Read the model definition and answer for the solid it produces. Units are mm, in the model's axes. Give positions to 0.01 mm unless a question says otherwise; leave off trailing zeros. Order: outer loops, then holes, each group sorted by start corner. A loop starts at its lowest first (then second) coordinate and runs counter-clockwise, first axis right, second up. Notation, with made-up numbers: (21.5, 76) -> (38.5, 76) arc R20 cw to (38.5, 94) -> close; hole circle Ø5 at (-17.5, -37). An arc over 180 degrees is marked (long way). One line per question, with ' | ' between items. Start each with the question number.
Autodesk Inventor part; units mm, degrees
ref_plane "Work Plane1" through (0, 0, 4) normal (0, 0, 1) x (1, 0, 0)
ref_plane "Work Plane3" through (0, 0, -1) normal (0, 0, 1) x (1, 0, 0)
ref_plane "Work Plane4" through (0, 0, 0) normal (0, 0, -1) x (-1, 0, 0)
sketch "Sketch1" plane through (0, 0, 0) normal (0, 0, 1) x (1, 0, 0)
  circle A0 centre (0, 0) radius 55
  dimension "d0" = 110
extrude "Extrusion1" add sketch "Sketch1" along normal blind 3
ref_plane "Work Plane1" through (0, 0, 4) normal (0, 0, 1) x (1, 0, 0)
sketch "Sketch2" plane through (0, 0, 4) normal (0, 0, 1) x (1, 0, 0)
  line L0 (-6.5, 6) -> (6.5, 6)
  line L1 (6.5, 6) -> (6.5, -18)
  line L2 (-6.5, -18) -> (-6.5, 6)
  circle A0 centre (-35.532, 35.532) radius 1.5
  circle A1 centre (-35.532, -35.532) radius 1.5
  circle A2 centre (35.532, -35.532) radius 1.5
  circle A3 centre (35.532, 35.532) radius 1.5
  line L3 (-6.5, -18) -> (6.5, -18)
  circle A4 centre (0, 8.5) radius 1
  circle A5 centre (0, -19.528) radius 1.9565
  point P0 (0, 0)
  point P1 (0, 6)
  point P2 (0, -13.848)
  dimension "d4" = 13
  dimension "d7" = 3
  dimension "d8" = 3
  dimension "d9" = 3
  dimension "d10" = 3
  dimension "d15" = 35.532
  dimension "d16" = 35.532
  dimension "d17" = 35.532
  dimension "d18" = 35.532
  dimension "d19" = 35.532
  dimension "d20" = 35.532
  dimension "d21" = 35.532
  dimension "d22" = 35.532
  dimension "d138" = 6
  dimension "d139" = 24
  dimension "d140" = 2
  dimension "d141" = 2.5
  dimension "d142" = 1.528
extrude "Extrusion2" cut sketch "Sketch2" against normal blind 4 contours L0 L1 L3 A5 L2 | A5 L3 picked at (0, -17.8572)
ref_plane "Work Plane2" through (0, 0, 3) normal (0, 0, 1) x (1, 0, 0)
sketch "Sketch3" plane through (0, 0, 3) normal (0, 0, 1) x (1, 0, 0)
  circle A0 centre (-35.577, 35.5342) radius 2.5
  circle A1 centre (-35.5225, -35.5931) radius 2.5
  circle A2 centre (35.5095, -35.5931) radius 2.5
  circle A3 centre (35.5095, 35.4262) radius 2.5
  point P0 (0, 0)
ref_plane "Work Plane3" through (0, 0, -1) normal (0, 0, 1) x (1, 0, 0)
ref_plane "Work Plane4" through (0, 0, 0) normal (0, 0, -1) x (-1, 0, 0)
sketch "Sketch5" plane through (0, 0, 0) normal (0, 0, -1) x (-1, 0, 0)
  line L0 (-9.906, 9.652) -> (9.906, 9.652)
  line L1 (9.906, 9.652) -> (9.906, -30.226)
  line L2 (9.906, -30.226) -> (-9.906, -30.226)
  line L3 (-9.906, -30.226) -> (-9.906, 9.652)
  circle A0 centre (-35.532, 35.532) radius 1.5
  circle A1 centre (-35.532, -35.532) radius 1.5
  circle A2 centre (35.532, -35.532) radius 1.5
  circle A3 centre (35.532, 35.532) radius 1.5
  circle A4 centre (-5.08, 13.462) radius 1
  circle A5 centre (5.08, 13.462) radius 1
  circle A6 centre (-5.08, -34.036) radius 1
  circle A7 centre (5.08, -34.036) radius 1
  point P0 (0, 0)
  point P1 (0, 0)
  point P2 (0, 9.652)
  point P3 (0, -30.226)
  dimension "d53" = 19.812
  dimension "d54" = 39.878
  dimension "d55" = 9.652
  dimension "d56" = 3
  dimension "d57" = 3
  dimension "d58" = 3
  dimension "d59" = 3
  dimension "d60" = 2
  dimension "d61" = 2
  dimension "d62" = 2
  dimension "d63" = 2
  dimension "d64" = 35.532
  dimension "d65" = 35.532
  dimension "d66" = 35.532
  dimension "d67" = 35.532
  dimension "d68" = 35.532
  dimension "d69" = 35.532
  dimension "d70" = 35.532
  dimension "d71" = 35.532
  dimension "d72" = 10.16
  dimension "d73" = 10.16
  dimension "d74" = 3.81
  dimension "d75" = 3.81
  dimension "d76" = 3.81
  dimension "d77" = 3.81
  dimension "d78" = 30.226
  dimension "d79" = 5.08
  dimension "d80" = 5.08
  dimension "d81" = 5.08
  dimension "d82" = 5.08
hole "Hole1" at (35.532, 35.532, 0) at (-35.532, 35.532, 0) at (35.532, -35.532, 0) at (-35.532, -35.532, 0) direction (0, 0, 1) diameter 2.459 depth 4 tip angle 118
ref_plane "Work Plane5" through (0, 0, 0) normal (0, 0, -1) x (-1, 0, 0)
fillet "Fillet1" radius 0.4125 4 edges at (6.5, -18, 1.5) (-6.5, -18, 1.5) (6.5, 6, 1.5) (-6.5, 6, 1.5)
ref_plane "Work Plane6" through (0, 0, 0) normal (0, 0, -1) x (-1, 0, 0)
ref_plane "Work Plane7" through (0, 0, 3) normal (0, 0, 1) x (1, 0, 0)
sketch "Sketch8" plane through (0, 0, 3) normal (0, 0, 1) x (1, 0, 0)
  circle A0 centre (0, -19.528) radius 1
  circle A1 centre (0, 8.5) radius 1
  line L0 (6.0875, -18) -> (-6.0875, -18)
  line L1 (-6.0875, 6) -> (6.0875, 6)
  point P0 (0, 0)
  point P1 (0, -18)
  point P2 (0, -18)
  dimension "d144" = 2
  dimension "d145" = 2
  dimension "d146" = 1.528
  dimension "d147" = 2.5
hole "Hole3" at (0, 8.5, 3) at (0, -19.528, 3) direction (0, 0, -1) diameter 1.567 depth 6.3 tip angle 118
properties part number "bottom-plate"
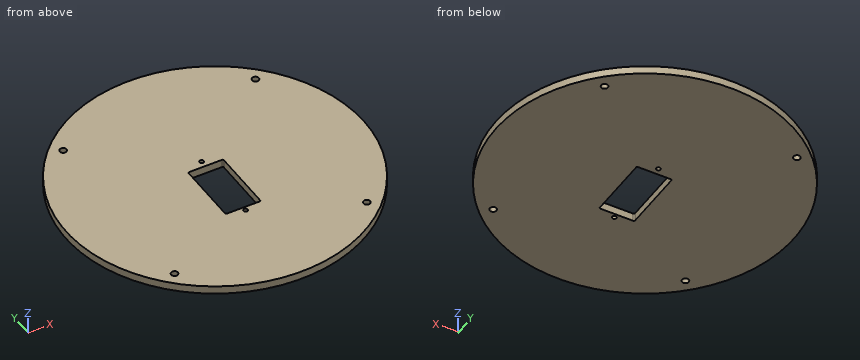
Q1. A cutting plane is placed at B-B, the plane x = -3. Determine the outline of the cut face in (y, z).
Q2. A cutting plane is placed at C-C, the plane z = 2.15. Determine the outline of the cut face in (x, y) (1 decimal).
Q3. A cutting plane is placed at D-D, the plane y = -30. Determine the outline of the cut face in (x, z).
Q4. Find the intervals of material crossed by line 1 (Y direction, x = 0, z = 0.9); line 2 (X direction, y = 36, z = 2.55); line 3 (Y direction, x = -34.5, z = 1.05), in increasing order.
Q5. Given P1, Ø1.5, axis at y = -2.5, z = 1.5, coming from the +X side; P2, Ø1.5, axis at y = -3, z = 2, coming from the -X side, each flat-ended and moving along its own axis, determine where each tip first touches the part or whether it passes through.
Q6. A cutting plane is placed at A-A, the plane y = 0. Determine the outline of the cut face in (x, z), then the cut area to 3 significant figures.
Geometry results:
1) outline: (-54.92, 0) -> (-18, 0) -> (-18, 3) -> (-54.92, 3) -> close; (6, 0) -> (54.92, 0) -> (54.92, 3) -> (6, 3) -> close
2) outline: circle Ø110 at (0, 0); hole circle Ø2.5 at (-35.5, -35.5); hole circle Ø2.5 at (-35.5, 35.5); hole (-6.5, -17.6) arc R0.4 ccw to (-6.1, -18) -> (6.1, -18) arc R0.4 ccw to (6.5, -17.6) -> (6.5, 5.6) arc R0.4 ccw to (6.1, 6) -> (-6.1, 6) arc R0.4 ccw to (-6.5, 5.6) -> close; hole circle Ø1.6 at (0, -19.5); hole circle Ø1.6 at (0, 8.5); hole circle Ø2.5 at (35.5, -35.5); hole circle Ø2.5 at (35.5, 35.5)
3) outline: (-46.1, 0) -> (46.1, 0) -> (46.1, 3) -> (-46.1, 3) -> close
4) line 1: -55 to -20.31, -18.74 to -18, 6 to 7.72, 9.28 to 55 | line 2: -41.58 to -36.67, -34.4 to 34.4, 36.67 to 41.58 | line 3: -42.83 to -36.2, -34.86 to 34.86, 36.2 to 42.83
5) P1: x = 54.97 | P2: x = -54.95
6) outline: (-55, 0) -> (-6.5, 0) -> (-6.5, 3) -> (-55, 3) -> close; (6.5, 0) -> (55, 0) -> (55, 3) -> (6.5, 3) -> close | area: 291 mm²
